Could you check a few things on this model? Use its own coordinates, in mm. Coordinates: 2 decimals unless noted, no trailing zeros. Order: outer loops, then holes, each group sorted by start corner. A loop starts at its lowest first (then second) coordinate and runs counter-clockwise, first axis right, second up. Notation, with made-up numbers: (49.5, 0) - (94.5, 0) arc R33 ccw to (94.5, 28) - close; hole circle Ø5 at (-36, 73). An arc over 180 degrees is marked (long way). One line per item, written item: value.
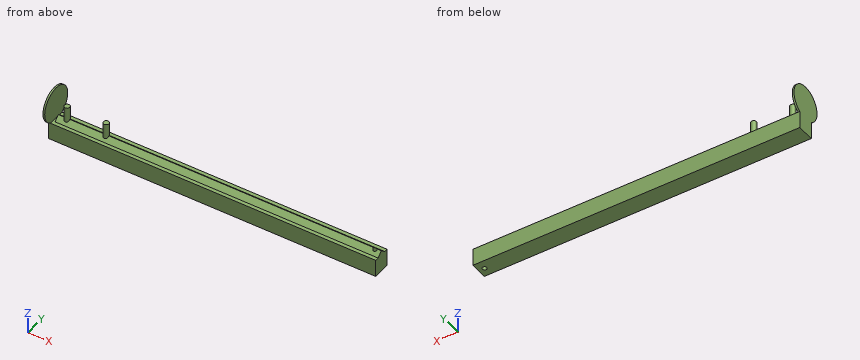
from build123d import *

# Parameters (mm, degrees)
F0_W          = 508
F0_H          = 25.4
F1_DEPTH      = 25.4
F3_DEPTH      = 508.001
F4_R          = 3.96875
F4_R_2        = 3.9751
F5_DEPTH      = 50.8
F6_R          = 3.175
F7_DEPTH      = 84.328
F7_DEPTH_BACK = 61.468
F9_DEPTH      = 25.4
F10_DEPTH     = 148.59
F11_W         = 25.4
F11_H         = 25.4
F12_DEPTH     = 3.175
F13_W         = 25.4
F13_H         = 25.4
F14_DEPTH     = 2.54


with BuildPart() as f1:
    # F0 (on Top) → F1 (new body)
    with BuildSketch(Plane.XY):
        with Locations((224.1236992961, 2.1686004475)):
            Rectangle(F0_W, F0_H)
    extrude(amount=F1_DEPTH)

    # F2 (on face) → F3 (join, through all)
    with BuildSketch(Plane(origin=(-29.8763007039, 0, 0), x_dir=(0, -1, 0), z_dir=(-1, 0, 0))):
        Polygon((-2.1686004475, 25.4), (-2.1686004475, 31.75), (-9.5885356279, 25.4), align=None)
        Polygon((5.251334733, 25.4), (-2.1686004475, 31.75), (-2.1686004475, 25.4), align=None)
    extrude(amount=-F3_DEPTH)

    # F4 (on Top) → F5 (join)
    with BuildSketch(Plane.XY):
        with Locations((-17.1763007039, 2.2061855998)):
            Circle(F4_R)
        with Locations((39.9736992961, 2.2061855998)):
            Circle(F4_R_2)
    extrude(amount=F5_DEPTH)

    # F6 (on Top) → F7 (cut, two sides)
    with BuildSketch(Plane.XY) as f7_sk:
        with Locations((433.6736992961, 2.1686004475)):
            Circle(F6_R)
    extrude(amount=F7_DEPTH, mode=Mode.SUBTRACT)
    extrude(f7_sk.sketch, amount=-F7_DEPTH_BACK, mode=Mode.SUBTRACT)


with BuildPart() as f9:
    # F8 (on Top) → F9 (new body)
    with BuildSketch(Plane.XY):
        Polygon((487.5240470482, 27.3656504085), (442.0609761506, 27.3656504085), (442.7554455138, -23.4296024435), (487.5240470482, -22.8175290615), align=None)
    extrude(amount=F9_DEPTH)


with BuildPart() as f10_tool:
    # F8 (on Top) → F10 (new body)
    with BuildSketch(Plane.XY):
        Polygon((487.5240470482, 27.3656504085), (442.0609761506, 27.3656504085), (442.7554455138, -23.4296024435), (487.5240470482, -22.8175290615), align=None)
    extrude(amount=F10_DEPTH)


with BuildPart() as f1_1:
    add(f1.part)

    # F10: cut by f10_tool
    add(f10_tool.part, mode=Mode.SUBTRACT)

    # F11 (on face) → F12 (join)
    with BuildSketch(Plane(origin=(-29.8763007039, 0, 0), x_dir=(0, -1, 0), z_dir=(-1, 0, 0))):
        with Locations((-2.1686004475, 12.7)):
            Rectangle(F11_W, F11_H)
    extrude(amount=F12_DEPTH)

    # F13 (on face) → F14 (join)
    with BuildSketch(Plane(origin=(-33.0513007039, 0, 0), x_dir=(0, -1, 0), z_dir=(-1, 0, 0))):
        with BuildLine():
            ThreePointArc((10.5313995525, 25.4), (-2.1686004475, 72.7970452561), (-14.8686004475, 25.4))
            Line((-14.8686004475, 25.4), (10.5313995525, 25.4))
        make_face()
        with Locations((-2.1686004475, 12.7)):
            Rectangle(F13_W, F13_H)
    extrude(amount=F14_DEPTH)


with BuildPart() as f9_1:
    add(f9.part)

    # F10: cut by f10_tool
    add(f10_tool.part, mode=Mode.SUBTRACT)


solid = f1_1.part
Item 1: I'm going to push flat-ended pins straight in: pin 1 Ø5 at (y, z) = (4, 17.5) entering from +X; pin 2 Ø2 at (x, z) = (297.5, 25.5) entering from -Y; pin 3 Ø4 at (x, y) = (356.5, 9.5) entering from +Z. Where does each tip first touch, or does it pass through?
Conclusion:
pin 1: x = 442.41
pin 2: y = -10.53
pin 3: z = 27.19
Item 2: I want a section at C-C on z = 36.5. Please give me the cut outline in (x, y), then the cut area to 3 significant figures.
Conclusion:
outline: (-35.59, -20.78) - (-33.05, -20.78) - (-33.05, 25.11) - (-35.59, 25.11) - close; circle Ø7.94 at (-17.18, 2.21); circle Ø7.95 at (39.97, 2.21)
area: 216 mm²
Item 3: I want a section at A-A on z = 19. Please give me the cut outline in (x, y) (3 decimals).
Conclusion:
outline: (-35.591, -10.531) - (442.579, -10.531) - (442.232, 14.869) - (-35.591, 14.869) - close; hole circle Ø6.35 at (433.674, 2.169)
Item 4: I want a section at B-B on x = 408. Please give me the cut outline in (y, z), then the cut area to 3 significant figures.
Conclusion:
outline: (-10.53, 0) - (14.87, 0) - (14.87, 25.4) - (9.59, 25.4) - (2.17, 31.75) - (-5.25, 25.4) - (-10.53, 25.4) - close
area: 692 mm²
Item 5: I want a section at D-D on y = 21. Please give me the cut outline in (x, z).
Conclusion:
outline: (-35.59, 30.35) - (-33.05, 30.35) - (-33.05, 64.44) - (-35.59, 64.44) - close
Item 6: If I drill on probe 1 along Y at (x, z) = (113.5, 4.5); probe 2 along X at (y, z) = (-2, 62.5); probe 3 along Z at (x, y) = (233.5, -10), over which ranges is the centre line in solid material (lowest first)?
Conclusion:
probe 1: -10.53 to 14.87
probe 2: -35.59 to -33.05
probe 3: 0 to 25.4
